Model file for the job. Use its own axes, mm. A direction names the side the tool comes from. Coordinates: 2 decimals unless noted, no trailing zeros. Write each loop counter-clockwise with the first axis right and the second up, starting at its lowest first coordinate (ties: lowest second). Pieces come first, ordered by that corner, then holes. Notation, with made-up numbers: (-22, -17.5) - (-4, -17.5) arc R26 ccw to (-4, 12.5) - close; hole circle Ø7 at (22, 43.5). An arc over 180 degrees is marked (long way). Put each result on its own line as item: value. Start each with the question number.
1. Saw through at C-C, the plane y = 46. Write the cut outline in (x, z), plus the area to 3 significant figures.
2. Saw through at A-A, the plane z = 0. Write the cut outline in (x, y).
3. Drill centre lines: L1, parallel to Z at x = 0, y = 27.5; L2, parallel to Y at x = 42, z = 33.5. Where is each one in solid material? Low to high. Write a range as from..to.
4. Drop flat-ended pins along their axis: P1, Ø8, axis at y = 47, z = 32, coming from the -X side; P2, Ø2, axis at x = 42.5, z = 43.5, coming from the +Y side; P3, Ø1, axis at y = 7, z = 15, coming from the +X side. Give the stop position or say it passes through.
5. Which spindle directions (+Z, -Z, +X, -X, +Y, -Y) get a long thin tool onto all of the face, cutting with end or side? Do faces 1 (the face through (-1, 5, -1)), 2 (the face through (-41, 55, -19)). Say none if no direction does.
6. Saw through at B-B, the plane x = 0. Write the cut outline in (y, z).
7. Saw through at D-D, the plane z = -48.5. Write the cut outline in (x, y), plus the area to 3 significant figures.
8. Pull direction Z, two halves, no side cores. Call faces 3 (the face through (20.765, 29.65, 39.923)), 4 (the face through (47.69, 29.65, -15.02)), 5 (the face through (-23, 5, -45)): released by +Z, released by -Z, zero draft, split by the parting line, or undercut.
```python
from build123d import *

# Parameters (mm, degrees)
SKETCH1_R           = 60
BOSS_EXTRUDE1_DEPTH = 5
SKETCH2_R           = 50
SKETCH2_R_2         = 45
BOSS_EXTRUDE2_DEPTH = 50


with BuildPart() as part:
    # Sketch1 → Boss-Extrude1 (new body)
    with BuildSketch(Plane(origin=(0, 0, 0), x_dir=(1, 0, 0), z_dir=(0, 1, 0))):
        Circle(SKETCH1_R)
    extrude(amount=BOSS_EXTRUDE1_DEPTH)

    # Sketch2 → Boss-Extrude2 (add)
    with BuildSketch(Plane(origin=(0, 5, 0), x_dir=(1, 0, 0), z_dir=(0, 1, 0))):
        Circle(SKETCH2_R)
        Circle(SKETCH2_R_2, mode=Mode.SUBTRACT)
    extrude(amount=BOSS_EXTRUDE2_DEPTH)


solid = part.part
```
Final values:
1. outline: circle Ø100 at (0, 0); hole circle Ø90 at (0, 0)
1. area: 1,490 mm²
2. outline: (-60, 0) - (60, 0) - (60, 5) - (50, 5) - (50, 55) - (45, 55) - (45, 5) - (-45, 5) - (-45, 55) - (-50, 55) - (-50, 5) - (-60, 5) - close
3. L1: z = -50..-45, 45..50
3. L2: y = 0..5
4. P1: stops at x = -41.42
4. P2: stops at y = 5
4. P3: stops at x = 47.85
5. face 1: +Y
5. face 2: +Z, -Z, +X, -X, +Y
6. outline: (0, -60) - (5, -60) - (5, -50) - (55, -50) - (55, -45) - (5, -45) - (5, 45) - (55, 45) - (55, 50) - (5, 50) - (5, 60) - (0, 60) - close
7. outline: (-35.32, 0) - (35.32, 0) - (35.32, 5) - (12.16, 5) - (12.16, 55) - (-12.16, 55) - (-12.16, 5) - (-35.32, 5) - close
7. area: 1,570 mm²
8. face 3: undercut
8. face 4: split by the parting line
8. face 5: zero draft
